Here's how the part is built. I have some questions about the finished solid (model axes, mm). A direction names the side the tool comes from. Round coordinates to 2 decimals unless told otherwise and drop trailing zeros. Write each loop counter-clockwise with the first axis right and the second up, starting at its lowest first coordinate (ties: lowest second). Pieces come first, ordered by that corner, then holes. Notation, with made-up numbers: (51, 77.25) - (97, 77.25) arc R24 cw to (97, 87.25) - close; hole circle Ø3 at (30, -20). An arc over 180 degrees is marked (long way). One line per item, written item: value. Start each with the question number.
Item 1: For faces 1 (the face through (28, 33, 2)), 2 (the face through (-56.874, 42.69, 1.521)), 3 (the face through (30, -41, 1)), which set-ups out of +Z, -Z, +X, -X, +Y, -Y let a thin tool reach every point of the face, with its end or its side?
Item 2: For P1, Ø1.4, axis at x = -50, y = 37.5, coming from the +Z side; P2, Ø1.5, axis at y = 42.5, z = 1.5, coming from the +X side; P3, Ø0.9, axis at x = 10, z = 1, coming from the +Y side; P4, Ø1.5, axis at y = -42, z = 2, coming from the +X side, each with a flat end and sliding along its axis, tell me the tip position at first contact or that it passes through.
Item 3: Imagine slicing it at D-D, the plane y = -19. Please give me the cut outline in (x, z).
Item 4: Imagine slicing it at B-B, the plane z = 0.85. Count the separate pieces of the cut face and the enclosed holes in it, then the cut area to 3 significant figures.
Item 5: Imagine slicing it at C-C, the plane x = -11. Please give me the cut outline in (y, z), then the cut area to 3 significant figures.
Item 6: Thinking about a two-plate mould opening in X: for faces 4 (the face through (-1, 1, 3)), 5 (the face through (0, 32, 1)), 6 (the face through (-29, -34, 2)), 7 (the face through (75, 0, 1)), which applies, released by +X, released by -X, zero draft, split by the parting line, or undercut?
Item 7: If I drill on line 1 (X direction, y = 37.5, z = 1.75); line 2 (Y direction, x = 50, z = 2.1); line 3 (X direction, y = -34, z = 2.45), over which ranges is the centre line in solid material (lowest first)?
Item 8: Imagine slicing it at A-A, the plane y = 35. Please give me the cut outline in (x, z), then the cut area to 3 significant figures.
```python
from build123d import *

# Parameters (mm, degrees)
BOSS_EXTRUDE1_DEPTH = 3
FILLET1_R           = 39
FILLET3_R           = 5
SKETCH7_R           = 0.75
CUT_EXTRUDE2_DEPTH  = 3
SKETCH8_R           = 0.75
CUT_EXTRUDE3_DEPTH  = 91.182696374


with BuildPart() as part:
    # Sketch1 → Boss-Extrude1 (new body)
    with BuildSketch(Plane.XY):
        Polygon((-30, 50), (-55, 50), (-55, -50), (-30, -50), (-30, -32), (30, -32), (30, -50), (55, -50), (55, 50), (30, 50), (30, 32), (-30, 32), align=None)
        with BuildLine():
            Line((-55, -50), (-55, 50))
            ThreePointArc((-55, 50), (-75, 0), (-55, -50))
        make_face()
        with BuildLine():
            ThreePointArc((55, -50), (75, 0), (55, 50))
            Line((55, 50), (55, -50))
        make_face()
    extrude(amount=BOSS_EXTRUDE1_DEPTH)

    # Fillet1
    fillet1_edges = [part.edges().sort_by_distance(p)[0] for p in [
        (-55, 50, 1.5),
        (55, 50, 1.5),
        (55, -50, 1.5),
        (-55, -50, 1.5),
    ]]
    fillet(fillet1_edges, radius=FILLET1_R)

    # Fillet3
    fillet3_edges = [part.edges().sort_by_distance(p)[0] for p in [
        (30, -50, 1.5),
        (-30, -50, 1.5),
        (30, 50, 1.5),
        (-30, 50, 1.5),
        (30, 32, 1.5),
        (-30, 32, 1.5),
        (-30, -32, 1.5),
        (30, -32, 1.5),
    ]]
    fillet(fillet3_edges, radius=FILLET3_R)

    # Sketch7 → Cut-Extrude2 (cut)
    with BuildSketch(Plane.XY.offset(3)):
        with Locations((-50, 37.5)):
            Circle(SKETCH7_R)
        with Locations((-50, -37.5)):
            Circle(SKETCH7_R)
        with Locations((50, -37.5)):
            Circle(SKETCH7_R)
        with Locations((50, 37.5)):
            Circle(SKETCH7_R)
    extrude(amount=-CUT_EXTRUDE2_DEPTH, mode=Mode.SUBTRACT)

    # Sketch8 → Cut-Extrude3 (cut, through all)
    with BuildSketch(Plane.XY.offset(3)):
        with Locations((-66.83099976, 8)):
            Circle(SKETCH8_R)
        with Locations((-66.83099976, -8)):
            Circle(SKETCH8_R)
        with Locations(Location((66.83099976, -8, 0), (0, 0, 180))):
            Circle(SKETCH8_R)
        with Locations(Location((66.83099976, 8, 0), (0, 0, 180))):
            Circle(SKETCH8_R)
    extrude(amount=-CUT_EXTRUDE3_DEPTH, mode=Mode.SUBTRACT)


solid = part.part
```
Values follow:
1. face 1: +Z, -Z, +Y
1. face 2: +Z, -Z, -X, +Y
1. face 3: +Z, -Z, -Y
2. P1: passes through
2. P2: stops at x = 58.13
2. P3: stops at y = 32
2. P4: stops at x = 58.76
3. outline: (-72.47, 0) - (72.47, 0) - (72.47, 3) - (-72.47, 3) - close
4. separate pieces: 1
4. enclosed holes: 8
4. area: 11,200 mm^2
5. outline: (-32, 0) - (32, 0) - (32, 3) - (-32, 3) - close
5. area: 192 mm^2
6. face 4: zero draft
6. face 5: undercut
6. face 6: undercut
6. face 7: released by +X
7. line 1: x = -62.76 to -50.75, -49.25 to -30, 30 to 49.25, 50.75 to 62.76
7. line 2: y = -46.63 to -38.25, -36.75 to 36.75, 38.25 to 46.63
7. line 3: x = -65.64 to -29, 29 to 65.64
8. outline: (-64.88, 0) - (-29.58, 0) - (-29.58, 3) - (-64.88, 3) - close; (29.58, 0) - (64.88, 0) - (64.88, 3) - (29.58, 3) - close
8. area: 212 mm^2
